Input: part model. Units: mm. Frame: model coordinates. Face numbers are marked on the shaded views. A direction names the side the tool comes from. Coordinates: 2 decimals unless noted, no trailing zeros. Write each loop counter-clockwise with the first axis right and the second up, starting at its lowest first coordinate (ties: lowest second). Pieces come first, ordered by that corner, then holes. Notation, with made-up numbers: (52.5, -39.5) - (95.5, -39.5) arc R20 cw to (95.5, -25.5) - close; hole circle Ø4 at (53.25, -16.75). An arc over 180 degrees is marked (long way). Use a Markdown table: item, result. Add a question column.
Q1. Mould query, pull axis X, two halves, no side actions, for the marked faces 3, 4, 5 and 6. Classes: released by +X, released by -X, zero draft, split by the parting line, or undercut.
Q2. Section query C-C (z = 2.25). Return the cut outline in (x, y) (3 decimals).
Q3. Material intervals for probe 1 along X at (y, z) = (0.25, 2.5); probe 2 along Y at (x, z) = (-4, 2.5) (3 decimals); probe 3 along Y at (x, z) = (2.5, 0.9) (3 decimals), sorted ascending. Write a range as from..to.
Q4. Section query A-A (x = 0.25). Return the cut outline in (y, z) (3 decimals), then the cut area to 3 significant figures.
Q5. Section query D-D (x = 5.25). Return the cut outline in (y, z) (3 decimals).
Q6. Section query B-B (y = -1.5). Return the cut outline in (x, z).
Q7. Set-up query: the marked faces 1 and 2. Return all of +Z, -Z, +X, -X, +Y, -Y with unobstructed straight access to the full face (end or side cutting, diameter ignored); none if empty.
from build123d import *

# Parameters (mm, degrees)
F1_DEPTH = 2
F3_DEPTH = 1
F4_DEPTH = 1


with BuildPart() as f1:
    # F0 (on Top) → F1 (new body)
    with BuildSketch(Plane.XY):
        with BuildLine():
            ThreePointArc((10.22, 4.625), (9.9271067812, 5.3321067812), (9.22, 5.625))
            Line((9.22, 5.625), (-9.22, 5.625))
            ThreePointArc((-9.22, 5.625), (-9.9271067812, 5.3321067812), (-10.22, 4.625))
            Line((-10.22, 4.625), (-10.22, -4.625))
            ThreePointArc((-10.22, -4.625), (-9.9271067812, -5.3321067812), (-9.22, -5.625))
            Line((-9.22, -5.625), (9.22, -5.625))
            ThreePointArc((9.22, -5.625), (9.9271067812, -5.3321067812), (10.22, -4.625))
            Line((10.22, -4.625), (10.22, 4.625))
        make_face()
        with BuildLine():
            Line((-7.22, 3.625), (7.22, 3.625))
            ThreePointArc((7.22, 3.625), (7.9271067812, 3.3321067812), (8.22, 2.625))
            Line((8.22, 2.625), (8.22, -2.625))
            ThreePointArc((8.22, -2.625), (7.9271067812, -3.3321067812), (7.22, -3.625))
            Line((7.22, -3.625), (-7.22, -3.625))
            ThreePointArc((-7.22, -3.625), (-7.9271067812, -3.3321067812), (-8.22, -2.625))
            Line((-8.22, -2.625), (-8.22, 2.625))
            ThreePointArc((-8.22, 2.625), (-7.9271067812, 3.3321067812), (-7.22, 3.625))
        make_face(mode=Mode.SUBTRACT)
    extrude(amount=F1_DEPTH)

    # F2 (on face) → F3 (join)
    with BuildSketch(Plane.XY.offset(2)):
        with BuildLine():
            Line((7.22, 3.625), (-7.22, 3.625))
            ThreePointArc((-7.22, 3.625), (-7.9271067812, 3.3321067812), (-8.22, 2.625))
            Line((-8.22, 2.625), (-8.22, -2.625))
            ThreePointArc((-8.22, -2.625), (-7.9271067812, -3.3321067812), (-7.22, -3.625))
            Line((-7.22, -3.625), (-4.1, -3.625))
            Line((-4.1, -3.625), (-4.1, -2.65))
            Line((-4.1, -2.65), (-6.6, -2.65))
            ThreePointArc((-6.6, -2.65), (-7.0242640687, -2.4742640687), (-7.2, -2.05))
            Line((-7.2, -2.05), (-7.2, 2.05))
            ThreePointArc((-7.2, 2.05), (-7.0242640687, 2.4742640687), (-6.6, 2.65))
            Line((-6.6, 2.65), (6.6, 2.65))
            ThreePointArc((6.6, 2.65), (7.0242640687, 2.4742640687), (7.2, 2.05))
            Line((7.2, 2.05), (7.2, -2.05))
            ThreePointArc((7.2, -2.05), (7.0242640687, -2.4742640687), (6.6, -2.65))
            Line((6.6, -2.65), (4.1, -2.65))
            Line((4.1, -2.65), (4.1, -3.625))
            Line((4.1, -3.625), (7.22, -3.625))
            ThreePointArc((7.22, -3.625), (7.9271067812, -3.3321067812), (8.22, -2.625))
            Line((8.22, -2.625), (8.22, 2.625))
            ThreePointArc((8.22, 2.625), (7.9271067812, 3.3321067812), (7.22, 3.625))
        make_face()
    extrude(amount=F3_DEPTH)

    # F4 (add): a face of the model
    f4_faces = [f1.faces().sort_by_distance(p)[0] for p in [
        (9.9866855984, 0, 2),
    ]]
    extrude(f4_faces, amount=F4_DEPTH)


solid = f1.part
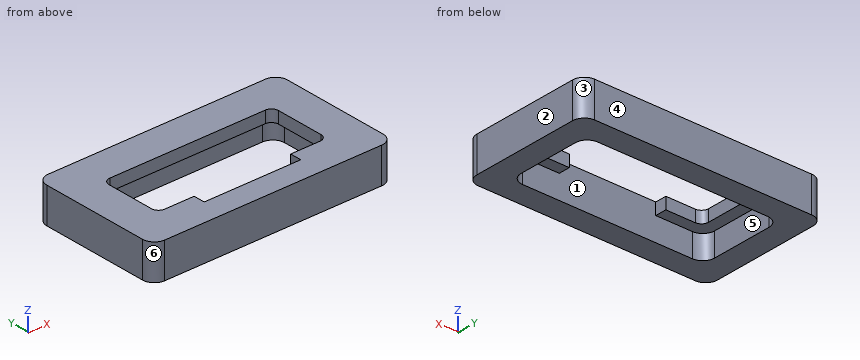
Values follow:
| question | item | result |
|---|---|---|
| 1 | face 3 | released by +X |
| 1 | face 4 | zero draft |
| 1 | face 5 | undercut |
| 1 | face 6 | released by -X |
| 2 | outline | (-10.22, -4.625) arc R1 ccw to (-9.22, -5.625) - (9.22, -5.625) arc R1 ccw to (10.22, -4.625) - (10.22, 4.625) arc R1 ccw to (9.22, 5.625) - (-9.22, 5.625) arc R1 ccw to (-10.22, 4.625) - close; hole (-7.2, -2.05) arc R0.6 ccw to (-6.6, -2.65) - (-4.1, -2.65) - (-4.1, -3.625) - (4.1, -3.625) - (4.1, -2.65) - (6.6, -2.65) arc R0.6 ccw to (7.2, -2.05) - (7.2, 2.05) arc R0.6 ccw to (6.6, 2.65) - (-6.6, 2.65) arc R0.6 ccw to (-7.2, 2.05) - close |
| 3 | probe 1 | -10.22..-7.2, 7.2..10.22 |
| 3 | probe 2 | -5.625..-3.625, 2.65..5.625 |
| 3 | probe 3 | -5.625..-3.625, 3.625..5.625 |
| 4 | outline | (-5.625, 0) - (-3.625, 0) - (-3.625, 3) - (-5.625, 3) - close; (2.65, 2) - (3.625, 2) - (3.625, 0) - (5.625, 0) - (5.625, 3) - (2.65, 3) - close |
| 4 | area | 13.0 mm2 |
| 5 | outline | (-5.625, 0) - (-3.625, 0) - (-3.625, 2) - (-2.65, 2) - (-2.65, 3) - (-5.625, 3) - close; (2.65, 2) - (3.625, 2) - (3.625, 0) - (5.625, 0) - (5.625, 3) - (2.65, 3) - close |
| 6 | outline | (-10.22, 0) - (-8.22, 0) - (-8.22, 2) - (-7.2, 2) - (-7.2, 3) - (-10.22, 3) - close; (7.2, 2) - (8.22, 2) - (8.22, 0) - (10.22, 0) - (10.22, 3) - (7.2, 3) - close |
| 7 | face 1 | -Z |
| 7 | face 2 | +Z, -Z, +X, +Y, -Y |
